Here's how the part is built. I have some questions about the finished solid (model axes, mm). Face numbers are marked on the shaded views. Give positions to 0.01 mm unless a question says otherwise; leave off trailing zeros. Write each loop counter-clockwise with the first axis right and the second up, starting at its lowest first coordinate (ties: lowest second). Pieces come first, ordered by that corner, then holes. Notation, with made-up numbers: (19, -10.75) -> (60, -10.75) arc R10 ccw to (60, -4.75) -> close; hole circle Ø9 at (-11, 7). An arc over 180 degrees is marked (long way). Return JSON: item names as keys, results as strings.
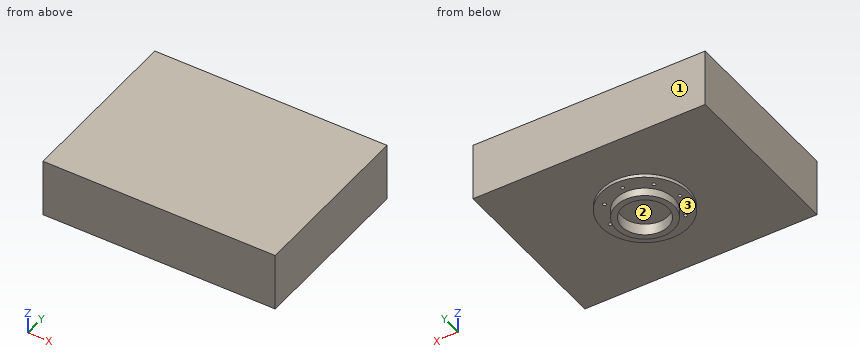
from build123d import *

# Parameters (mm, degrees)
SKETCH_1_R               = 37.5
EXTRUDE_1_DEPTH          = 3
SKETCH_2_R               = 25
CUT_EXTRUDE_1_DEPTH      = 3
SKETCH_3_R               = 1.5
CUT_EXTRUDE_2_DEPTH      = 13
PATTERN_CIRCULAR_1_COUNT = 8
EXTRUDE_2_DEPTH          = 5
EXTRUDE_2_DEPTH_BACK     = 10
SKETCH_4_R               = 25
SKETCH_4_R_2             = 20
SKETCH_6_W               = 200
SKETCH_6_H               = 150
EXTRUDE_3_DEPTH          = 50


with BuildPart() as part:
    # 草图1 → 凸台-拉伸1 (new body)
    with BuildSketch(Plane.XY):
        Circle(SKETCH_1_R)
    extrude(amount=EXTRUDE_1_DEPTH)

    # 草图2 → 切除-拉伸1 (cut)
    with BuildSketch(Plane(origin=(0, 0, 0), x_dir=(-1, 0, 0), z_dir=(0, 0, -1))):
        Circle(SKETCH_2_R)
    extrude(amount=-CUT_EXTRUDE_1_DEPTH, mode=Mode.SUBTRACT)

    # 草图3 → 切除-拉伸2 (cut)
    with BuildSketch(Plane.XY.offset(3)):
        with Locations((0, -30)):
            Circle(SKETCH_3_R)
    cut_extrude_2 = extrude(amount=-CUT_EXTRUDE_2_DEPTH, mode=Mode.SUBTRACT)

    # 阵列(圆周)1: 切除-拉伸2 ×8 about axis
    pattern_circular_1_axis = Axis((0, 0, 0), (0, 0, 1))
    for i in range(1, PATTERN_CIRCULAR_1_COUNT):
        add(cut_extrude_2.rotate(pattern_circular_1_axis, i * 360 / PATTERN_CIRCULAR_1_COUNT), mode=Mode.SUBTRACT)

    # 草图4 → 凸台-拉伸2 (add, two sides: drawn at the far end of the back side and taken through both)
    with BuildSketch(Plane.XY.offset(3).offset(-EXTRUDE_2_DEPTH_BACK)):
        with Locations(Location((0, 0, 0), (0, 0, 180))):
            Circle(SKETCH_4_R)
        Circle(SKETCH_4_R_2, mode=Mode.SUBTRACT)
    extrude(amount=EXTRUDE_2_DEPTH + EXTRUDE_2_DEPTH_BACK)

    # 草图6 → 凸台-拉伸3 (add)
    with BuildSketch(Plane.XY.offset(3)):
        Rectangle(SKETCH_6_W, SKETCH_6_H)
    extrude(amount=EXTRUDE_3_DEPTH)


solid = part.part
1. Suppose I cut it at B-B, the plane y = -53. List the corners of the cut face in (x, z) for me.
Taken from the geometry:
{"outline": "(-100, 3) -> (100, 3) -> (100, 53) -> (-100, 53) -> close"}
2. If we mould it in two halves opening along Y, with no side actions, what happens to the marked faces 1, 2 and 3? For each: released by +Y, released by -Y, zero draft, split by the parting line, or undercut.
Taken from the geometry:
{"face 1": "released by +Y", "face 2": "undercut", "face 3": "zero draft"}
3. If I drill on line 1 (Y direction, x = 0, z = -3); line 2 (Z direction, x = -8, y = -14.5); line 3 (Y direction, x = 4, z = -1), over which ranges is the centre line in solid material (lowest first)? Write a range as [from, to].
Taken from the geometry:
{"line 1": "y = [-25, -20], [20, 25]", "line 2": "z = [3, 53]", "line 3": "y = [-24.68, -19.6], [19.6, 24.68]"}
4. For pin 1 Ø5 at (x, y) = (21.21, 21.21) entering from -Z; pin 2 Ø1.8 at (x, y) = (-21.21, 21.21) entering from -Z; pin 3 Ø20 at (x, y) = (-7, 9.5) entering from -Z, each with a flat end and sliding along its axis, tell me the tip position at first contact or that it passes through.
Taken from the geometry:
{"pin 1": "stops at z = 0", "pin 2": "stops at z = 3", "pin 3": "stops at z = -7"}
5. Suppose I cut it at A-A, the plane x = 74. List the corners of the cut face in (y, z) for me.
Taken from the geometry:
{"outline": "(-75, 3) -> (75, 3) -> (75, 53) -> (-75, 53) -> close"}
